The listing builds one solid part. Answer for the finished solid, in the listing's coordinates (mm). A direction names the side the tool comes from. Round coordinates to 2 decimals unless told otherwise and drop trailing zeros. Loops run counter-clockwise (first coordinate to the right, second up) from the corner with the lowest first, then second, coordinate; pieces in that order, holes last. Notation, with made-up numbers: (-3, 26) -> (42, 26) arc R19 ccw to (42, 50) -> close; hole circle Ø10 at (53.25, -23.75). An arc over 180 degrees is marked (long way). Write each question's results on one line, items separated by ' | '. Start each with the question number.
from build123d import *
from OCP.BRepFilletAPI import BRepFilletAPI_MakeChamfer

# Parameters (mm, degrees)
SKETCH1_W               = 38
SKETCH1_H               = 55
BOSS_EXTRUDE1_DEPTH     = 20
CUT_EXTRUDE1_DEPTH      = 39.951893407
SKETCH3_R               = 2.25
CUT_EXTRUDE2_DEPTH      = 20
LPATTERN1_COUNT         = 3
LPATTERN1_PITCH         = 6
CHAMFER1_SIZE           = 12
SKETCH4_W               = 5
SKETCH4_H               = 8
BOSS_EXTRUDE2_DEPTH     = 10
FILLET1_R               = 4
SKETCH5_R               = 1.75
CUT_EXTRUDE3_DEPTH      = 58.010963858
FILLET1_OF_MIRROR1_R    = 4
CHAMFER2_SIZE           = 1
SKETCH6_R               = 7.5
CUT_EXTRUDE4_DEPTH      = 17
CUT_EXTRUDE5_DEPTH      = 46.345892868
CUT_EXTRUDE5_DEPTH_BACK = 46.345892868
SKETCH7_R               = 2
SKETCH8_W               = 7
SKETCH8_H               = 40
BOSS_EXTRUDE3_DEPTH     = 8
CHAMFER3_SIZE           = 15.045811723
CHAMFER3_SIZE_2         = 8


# Some blends are built 0.0001 mm under size
with BuildPart() as part:
    # Sketch1 → Boss-Extrude1 (new body)
    with BuildSketch(Plane.XY):
        Rectangle(SKETCH1_W, SKETCH1_H)
    extrude(amount=BOSS_EXTRUDE1_DEPTH)

    # Sketch2 → Cut-Extrude1 (cut, through all)
    with BuildSketch(Plane.XY.offset(20)):
        with BuildLine():
            Line((-12, -27.5), (12, -27.5))
            Line((12, -27.5), (12, -7.5))
            ThreePointArc((12, -7.5), (0, 4.5), (-12, -7.5))
            Line((-12, -7.5), (-12, -27.5))
        make_face()
    extrude(amount=-CUT_EXTRUDE1_DEPTH, mode=Mode.SUBTRACT)

    # Sketch3 → Cut-Extrude2 (cut)
    with BuildSketch(Plane.XZ.offset(27.5)):
        with Locations(Location((-15, 16, 0), (0, 0, 270))):
            Circle(SKETCH3_R)
        with Locations(Location((15, 16, 0), (0, 0, 270))):
            Circle(SKETCH3_R)
    cut_extrude2 = extrude(amount=-CUT_EXTRUDE2_DEPTH, mode=Mode.SUBTRACT)

    # LPattern1: Cut-Extrude2 ×3
    with Locations(*[(0, 0, -i * LPATTERN1_PITCH) for i in range(1, LPATTERN1_COUNT)]):
        add(cut_extrude2, mode=Mode.SUBTRACT)

    # Chamfer1
    chamfer1_edges = [part.edges().sort_by_distance(p)[0] for p in [
        (0, 27.5, 20),
    ]]
    chamfer(chamfer1_edges, length=CHAMFER1_SIZE)

    # Sketch4 → Boss-Extrude2 (add)
    with BuildSketch(Plane(origin=(0, 27.5, 0), x_dir=(1, 0, 0), z_dir=(0, 1, 0))):
        with Locations((-16.5, -4)):
            Rectangle(SKETCH4_W, SKETCH4_H)
    boss_extrude2 = extrude(amount=BOSS_EXTRUDE2_DEPTH)

    # Fillet1
    fillet1_edges = [part.edges().sort_by_distance(p)[0] for p in [
        (-16.5, 37.5, 0),
        (-16.5, 37.5, 8),
    ]]
    fillet(fillet1_edges, radius=FILLET1_R - 0.0001)  # a hair under: the kernel refuses the full size

    # Sketch5 → Cut-Extrude3 (cut, through all)
    with BuildSketch(Plane.ZY.offset(19)):
        with Locations((4, 33.5)):
            Circle(SKETCH5_R)
    cut_extrude3 = extrude(amount=-CUT_EXTRUDE3_DEPTH, mode=Mode.SUBTRACT)

    # Mirror1: Boss-Extrude2, Cut-Extrude3 across plane
    add(boss_extrude2.mirror(Plane(origin=(0, 0, 0), x_dir=(0, 0, 1), z_dir=(1, 0, 0))))
    add(cut_extrude3.mirror(Plane(origin=(0, 0, 0), x_dir=(0, 0, 1), z_dir=(1, 0, 0))), mode=Mode.SUBTRACT)

    # Fillet1 of Mirror1
    fillet1_of_mirror1_edges = [part.edges().sort_by_distance(p)[0] for p in [
        (16.5, 37.5, 0),
        (16.5, 37.5, 8),
    ]]
    fillet(fillet1_of_mirror1_edges, radius=FILLET1_OF_MIRROR1_R - 0.0001)  # a hair under: the kernel refuses the full size

    # Chamfer2
    # the kernel refuses this chamfer: 1 mm, written as the material it takes off along each edge
    with BuildSketch(Plane(origin=(-15, -27.5, 16), x_dir=(0, 0, -1), z_dir=(-1, 0, 0))) as chamfer2_piece_1:
        Polygon((2.25 + CHAMFER2_SIZE, 0), (2.25, -CHAMFER2_SIZE), (2.25, 0), align=None)
    revolve(axis=Axis((-15, -27.5, 16), (0, -1, 0)), mode=Mode.SUBTRACT)
    with BuildSketch(Plane(origin=(15, -27.5, 16), x_dir=(0, 0, -1), z_dir=(-1, 0, 0))) as chamfer2_piece_2:
        Polygon((2.25 + CHAMFER2_SIZE, 0), (2.25, -CHAMFER2_SIZE), (2.25, 0), align=None)
    revolve(axis=Axis((15, -27.5, 16), (0, -1, 0)), mode=Mode.SUBTRACT)
    with BuildSketch(Plane(origin=(-15, -27.5, 10), x_dir=(0, 0, -1), z_dir=(-1, 0, 0))) as chamfer2_piece_3:
        Polygon((2.25 + CHAMFER2_SIZE, 0), (2.25, -CHAMFER2_SIZE), (2.25, 0), align=None)
    revolve(axis=Axis((-15, -27.5, 10), (0, -1, 0)), mode=Mode.SUBTRACT)
    with BuildSketch(Plane(origin=(-15, -27.5, 4), x_dir=(0, 0, -1), z_dir=(-1, 0, 0))) as chamfer2_piece_4:
        Polygon((2.25 + CHAMFER2_SIZE, 0), (2.25, -CHAMFER2_SIZE), (2.25, 0), align=None)
    revolve(axis=Axis((-15, -27.5, 4), (0, -1, 0)), mode=Mode.SUBTRACT)
    with BuildSketch(Plane(origin=(15, -27.5, 10), x_dir=(0, 0, -1), z_dir=(-1, 0, 0))) as chamfer2_piece_5:
        Polygon((2.25 + CHAMFER2_SIZE, 0), (2.25, -CHAMFER2_SIZE), (2.25, 0), align=None)
    revolve(axis=Axis((15, -27.5, 10), (0, -1, 0)), mode=Mode.SUBTRACT)
    with BuildSketch(Plane(origin=(15, -27.5, 4), x_dir=(0, 0, -1), z_dir=(-1, 0, 0))) as chamfer2_piece_6:
        Polygon((2.25 + CHAMFER2_SIZE, 0), (2.25, -CHAMFER2_SIZE), (2.25, 0), align=None)
    revolve(axis=Axis((15, -27.5, 4), (0, -1, 0)), mode=Mode.SUBTRACT)

    # Sketch6 → Cut-Extrude4 (cut)
    with BuildSketch(Plane.XY.offset(20)):
        with Locations((0, 21.5)):
            Circle(SKETCH6_R)
    extrude(amount=-CUT_EXTRUDE4_DEPTH, mode=Mode.SUBTRACT)

    # Sketch7 → Cut-Extrude5 (cut, two sides: drawn at the far end of the back side and taken through both)
    with BuildSketch(Plane.XY.offset(3).offset(-CUT_EXTRUDE5_DEPTH_BACK)):
        with Locations((0, 21.5)):
            Circle(SKETCH7_R)
    extrude(amount=CUT_EXTRUDE5_DEPTH + CUT_EXTRUDE5_DEPTH_BACK, mode=Mode.SUBTRACT)

    # Sketch8 → Boss-Extrude3 (add)
    with BuildSketch(Plane(origin=(0, 0, 0), x_dir=(-1, 0, 0), z_dir=(0, 0, -1))):
        with Locations((-15.5, -7.5)):
            Rectangle(SKETCH8_W, SKETCH8_H)
        with Locations((15.5, -7.5)):
            Rectangle(SKETCH8_W, SKETCH8_H)
    extrude(amount=BOSS_EXTRUDE3_DEPTH)

    # Chamfer3
    chamfer3_edges_1 = [part.edges().sort_by_distance(p)[0] for p in [
        (-15.5, 12.5, -8),
    ]]
    chamfer3_side_1 = [part.faces().sort_by_distance(p)[0] for p in [
        (-15.5, 12.34, -8),
    ]]
    chamfer3_edges_2 = [part.edges().sort_by_distance(p)[0] for p in [
        (15.5, 12.5, -8),
    ]]
    chamfer3_side_2 = [part.faces().sort_by_distance(p)[0] for p in [
        (15.5, 12.34, -8),
    ]]
    chamfer3 = BRepFilletAPI_MakeChamfer(part.part.solid().wrapped)
    for e in chamfer3_edges_1:
        chamfer3.Add(CHAMFER3_SIZE - 0.0001, CHAMFER3_SIZE_2 - 0.0001, e.wrapped, chamfer3_side_1[0].wrapped)
    for e in chamfer3_edges_2:
        chamfer3.Add(CHAMFER3_SIZE - 0.0001, CHAMFER3_SIZE_2 - 0.0001, e.wrapped, chamfer3_side_2[0].wrapped)
    add(Compound.cast(chamfer3.Shape()), mode=Mode.REPLACE)  # a hair under: the kernel refuses the full size


solid = part.part
Item 1: Each of these flat-tipped pins is pushed along its axis until it touches: pin 1 Ø1.5 at (x, z) = (-8, 7.5) entering from +Y; pin 2 Ø1.3 at (x, z) = (-15.5, 10.5) entering from -Y; pin 3 Ø4 at (x, y) = (2.5, 12) entering from -Z; pin 4 Ø2.5 at (y, z) = (34.5, 5) entering from +X. Where does it stop, or does it pass through?
Item 2: The part is cut by section C-C, the plane z = 16. Give the vertices of the cut face in (x, y), plus the area to 3 significant figures.
Item 3: The part is cut by section B-B, the plane y = 21.5. Give the vertices of the cut face in (x, z).
Item 4: For faces 4 (the flat face through (12, -12, 6)), 5 (the flat face through (15, -7.5, 4)), 6 (the flat face through (0, 27.5, 2)), 7 (the flat face through (13.3, 21.4, 14.1)), determine the directions among +Z, -Z, +X, -X, +Y, -Y from which every point of the face is accessible in a straight line to the end or side of a thin tool.
Item 5: The part is cut by section A-A, the plane y = -14.5. Give the vertices of the cut face in (x, z).
Item 6: Determine the mould class of faces 1 (the cylindrical face through (13.004, -17.133, 2.962)), 2 (the flat face through (-15, -15, -8)), 3 (the flat face through (-17, 30, 8)) for opening direction Z: +Z half, -Z half, draft (parallel to the pull), parting line (faces both ways), or undercut.
Item 7: The part is cut by section D-D, the plane x = -9. Give the vertices of the cut face in (y, z), plus the area to 3 significant figures.
Item 8: Straight lines are drawn through the part: L1, parallel to X at y = -22, z = 4; L2, parallel to X at y = -21, z = 13.5; L3, parallel to Z at x = -4, y = 6. For each, find the intervals that lie inside material, in ascending order. Write a range as [from, to].
Report:
1) pin 1: stops at y = 27.5 | pin 2: stops at y = -7.5 | pin 3: stops at z = 0 | pin 4: stops at x = 19
2) outline: (-19, -27.5) -> (-18.25, -27.5) -> (-17.25, -26.5) -> (-17.25, -7.5) -> (-12.75, -7.5) -> (-12.75, -26.5) -> (-12, -27.25) -> (-12, -7.5) arc R12 cw to (12, -7.5) -> (12, -27.25) -> (12.75, -26.5) -> (12.75, -7.5) -> (17.25, -7.5) -> (17.25, -26.5) -> (18.25, -27.5) -> (19, -27.5) -> (19, 19.5) -> (7.23, 19.5) arc R7.5 cw to (-7.23, 19.5) -> (-19, 19.5) -> close | area: 839 mm2
3) outline: (-19, 0) -> (-2, 0) -> (-2, 3) -> (-7.5, 3) -> (-7.5, 14) -> (-19, 14) -> close; (2, 0) -> (19, 0) -> (19, 14) -> (7.5, 14) -> (7.5, 3) -> (2, 3) -> close
4) face 4: -Z, -Y | face 5: -Y | face 6: +Z, -Z, +Y | face 7: +Z, +X, -X, +Y
5) outline: (-19, -8) -> (-12, -8) -> (-12, 20) -> (-19, 20) -> close; (12, -8) -> (19, -8) -> (19, 20) -> (12, 20) -> close; hole circle Ø4.5 at (-15, 4); hole circle Ø4.5 at (-15, 10); hole circle Ø4.5 at (-15, 16); hole circle Ø4.5 at (15, 4); hole circle Ø4.5 at (15, 10); hole circle Ø4.5 at (15, 16)
6) face 1: undercut | face 2: -Z half | face 3: +Z half
7) outline: (0.44, 0) -> (27.5, 0) -> (27.5, 8) -> (15.5, 20) -> (0.44, 20) -> close | area: 469 mm2
8) L1: x = [-19, -17.25], [-12.75, -12], [12, 12.75], [17.25, 19] | L2: x = [-19, -12], [12, 19] | L3: z = [0, 20]
